CAD build for the part. Positions are in the model's coordinates, mm. A direction names the side the tool comes from. Round coordinates to 2 decimals unless told otherwise and drop trailing zeros. Write each loop counter-clockwise with the first axis right and the second up, starting at its lowest first coordinate (ties: lowest second). Pieces come first, ordered by that corner, then holes. Notation, with made-up numbers: (74.25, 4.5) - (113.25, 4.5) arc R24 ccw to (113.25, 23.5) - close; hole circle Ø1 at (33, -22.75). An arc over 180 degrees is marked (long way). Use one line per item in the form item = value. Start each with the question number.
Item 1: Band-saw the part on C-C, the plane y = 61. List the corners of the cut face in (x, z), and give its area (3 significant figures).
Item 2: Band-saw the part on B-B, the plane x = -68.5. List the corners of the cut face in (y, z), and give its area (3 significant figures).
Item 3: Tool access for faces 1 (the flat face through (-38, 50.8, -38)), 2 (the flat face through (0, 25, -64)), 3 (the flat face through (-165, 50.8, -38)): list every direction of +Z, -Z, +X, -X, +Y, -Y with a clear straight run to the whole face (end or side of a thin tool).
Item 4: Drill centre lines: L1, parallel to Z at x = -140, y = 60; L2, parallel to Y at x = -10, z = -25. Where is each one in solid material? Low to high.
Item 5: Pin check, flat tips, straight feed: pin 1 (23 mm diameter, centred on x = -167.5, y = 82, fed in from +Z); pin 2 (23 mm diameter, centred on x = -47, z = -25.5, fed in from +Y); pin 3 (3 mm diameter, centred on y = 47.5, z = -105, fed in from +X); pin 4 (1.5 mm diameter, centred on y = 84, z = -76.5, fed in from +X). Stop position of each tip, or through.
Autodesk Inventor part; units mm, degrees
ref_plane "YZ Plane" through (0, 0, 0) normal (1, 0, 0) x (0, 1, 0)
ref_plane "XZ Plane" through (0, 0, 0) normal (0, 1, 0) x (-1, 0, 0)
ref_plane "XY Plane" through (0, 0, 0) normal (0, 0, 1) x (1, 0, 0)
sketch "Sketch1" plane through (0, 0, 0) normal (0, 1, 0) x (-1, 0, 0)
  line L0 (0, 0) -> (203.2, 0)
  line L1 (203.2, 0) -> (203.2, -127)
  line L2 (203.2, -127) -> (0, -127)
  line L3 (0, -127) -> (0, 0)
  dimension "d0" = 203.2
  dimension "d1" = 127
extrude "Extrusion1" add sketch "Sketch1" along normal blind 50.8
sketch "Sketch2" plane through (0, 50.8, 0) normal (0, 1, 0) x (1, 0, 0)
  line L0 (-203.2, 127) -> (-203.2, 0)
  line L1 (-203.2, 76.2) -> (0, 76.2)
  line L2 (0, 76.2) -> (0, 127)
  line L3 (0, 127) -> (-203.2, 127)
  line L4 (-203.2, 127) -> (-203.2, 76.2)
  point P0 (0, 0)
  dimension "d4" = 50.8
  dimension "d13" = 203.2
extrude "Extrusion2" add sketch "Sketch2" along normal blind 76.2
chamfer "Chamfer1" distance 50.8 angle 56.31 1 edges at (0, 127, -101.6) measured on face at (-67.7333, 127, -110.0667)
sketch "Sketch3" plane through (0, 50.8, 0) normal (0, 1, 0) x (1, 0, 0)
  line L0 (0, 76.2) -> (-203.2, 76.2)
  line L1 (-127, 76.2) -> (-76.2, 76.2)
  line L2 (-76.2, 76.2) -> (-76.2, 0)
  line L3 (-76.2, 0) -> (-127, 0)
  line L4 (-127, 0) -> (-127, 76.2)
  line L5 (-203.2, 76.2) -> (-203.2, 0)
  point P0 (0, 0)
  dimension "d10" = 50.8
  dimension "d11" = 76.2
  dimension "d12" = 76.2
extrude "Extrusion3" add sketch "Sketch3" along normal blind 76.2
chamfer "Chamfer2" distance 76.2 angle 45 1 edges at (-101.6, 127, 0)
sketch "Sketch4" plane through (-0.0002, 50.7998, -127) normal (0.8321, 0.5547, 0) x (-0.5547, 0.8321, 0)
  point P0 (-42.2682, 127)
sketch "Sketch5" plane through (0, 127, 0) normal (0, 1, 0) x (1, 0, 0)
  point P0 (0, 0)
sketch "Sketch6" plane through (-50.8, 127, -127) normal (0.8321, 0.5547, 0) x (-0.5547, 0.8321, 0)
  point P0 (-133.8492, 127)
Determined:
q1.outline = (-203.2, -127) - (-6.8, -127) - (-6.8, -76.2) - (-76.2, -76.2) - (-76.2, -10.2) - (-127, -10.2) - (-127, -76.2) - (-203.2, -76.2) - close
q1.area = 13,300 mm²
q2.outline = (0, -127) - (127, -127) - (127, -76.2) - (50.8, -76.2) - (50.8, 0) - (0, 0) - close
q2.area = 10,300 mm²
q3.face_1 = +Z, +X, +Y
q3.face_2 = +Z, -Z, +X, +Y, -Y
q3.face_3 = +Z, -X, +Y
q4.L1 = -127 to -76.2
q4.L2 = 0 to 50.8
q5.pin_1 = -76.2
q5.pin_2 = 50.8
q5.pin_3 = 0
q5.pin_4 = -21.63
